Can you work these out from the model? Positions are in its coordinate system, mm. A direction names the side the tool comes from. Give positions to 0.01 mm unless a question says otherwise; leave off trailing zeros. Order: outer loops, then holes, each group sorted by start corner. A loop starts at its lowest first (then second) coordinate and runs counter-clockwise, first axis right, second up. Notation, with made-up numbers: (85, 71) -> (95, 71) arc R21 ccw to (95, 97) -> close; hole circle Ø9 at (-10, -13.5). An arc over 180 degrees is marked (long way). Answer as a JSON object with one key per item and string values.
```python
from build123d import *

# Parameters (mm, degrees)
SKETCH1_R              = 14.2875
BOSS_EXTRUDE1_DEPTH    = 3.175
SKETCH2_W              = 44.45
SKETCH2_H              = 3.175
BOSS_EXTRUDE2_DEPTH    = 50.8
FILLET1_R              = 2.54
CONVERT_SOLID1_START   = -22.225
CONVERT_SOLID1_DEPTH   = 44.45
CONVERT_SOLID1_2_DEPTH = 44.45
SKETCH7_R              = 2.413
CUT_EXTRUDE1_DEPTH     = 50.8


# Read off the part's stored shape, not the designer's step: Convert-Solid1
with BuildPart() as part:
    # Sketch1 → Boss-Extrude1 (new body)
    with BuildSketch(Plane.XY):
        with BuildLine():
            Line((-22.225, -46.491872792), (22.225, -46.491872792))
            Line((22.225, -46.491872792), (22.225, 43.951872792))
            ThreePointArc((22.225, 43.951872792), (21.481051224, 45.747924016), (19.685, 46.491872792))
            Line((19.685, 46.491872792), (-19.685, 46.491872792))
            ThreePointArc((-19.685, 46.491872792), (-21.481051224, 45.747924016), (-22.225, 43.951872792))
            Line((-22.225, 43.951872792), (-22.225, -46.491872792))
        make_face()
        with Locations((0, 22.596127208)):
            Circle(SKETCH1_R, mode=Mode.SUBTRACT)
    extrude(amount=BOSS_EXTRUDE1_DEPTH)

    # Sketch2 → Boss-Extrude2 (add)
    with BuildSketch(Plane(origin=(0, 0, 0), x_dir=(-1, 0, 0), z_dir=(0, 0, -1))):
        with Locations((0, -44.904372792)):
            Rectangle(SKETCH2_W, SKETCH2_H)
    extrude(amount=BOSS_EXTRUDE2_DEPTH)

    # Fillet1
    fillet1_edges = [part.edges().sort_by_distance(p)[0] for p in [
        (22.225, -44.904372792, -50.8),
        (-22.225, -44.904372792, -50.8),
    ]]
    fillet(fillet1_edges, radius=FILLET1_R)

    # Convert-Solid1 outline → Convert-Solid1 (cut)
    with BuildSketch(Plane.YZ.offset(CONVERT_SOLID1_START)):
        with BuildLine():
            ThreePointArc((-46.491872792, -3.81), (-44.446013659, 1.129140866), (-39.506872792, 3.175))
            Line((-39.506872792, 3.175), (-46.491872792, 3.175))
            Line((-46.491872792, 3.175), (-46.491872792, -3.81))
        make_face()
    extrude(amount=CONVERT_SOLID1_DEPTH, mode=Mode.SUBTRACT)

    # Convert-Solid1 2 outline → Convert-Solid1 2 (add)
    with BuildSketch(Plane.YZ.offset(CONVERT_SOLID1_START)):
        with BuildLine():
            ThreePointArc((-43.316872792, -3.81), (-42.200949628, -1.115923164), (-39.506872792, 0))
            Line((-39.506872792, 0), (-43.316872792, 0))
            Line((-43.316872792, 0), (-43.316872792, -3.81))
        make_face()
    extrude(amount=CONVERT_SOLID1_2_DEPTH)

    # Sketch7 → Cut-Extrude1 (cut)
    with BuildSketch(Plane(origin=(0, -43.316872792, 0), x_dir=(1, 0, 0), z_dir=(0, 1, 0))):
        with Locations(Location((-10.795, 39.37, 0), (0, 0, 180))):
            Circle(SKETCH7_R)
        with Locations(Location((10.795, 39.37, 0), (0, 0, 180))):
            Circle(SKETCH7_R)
        with Locations(Location((-10.795, 16.51, 0), (0, 0, 180))):
            Circle(SKETCH7_R)
        with Locations(Location((10.795, 16.51, 0), (0, 0, 180))):
            Circle(SKETCH7_R)
    extrude(amount=-CUT_EXTRUDE1_DEPTH, mode=Mode.SUBTRACT)


solid = part.part
```
1. For faces 1 (the face through (22.225, -14.9, 0.4)), 2 (the face through (0, 4, 0)), which set-ups out of +Z, -Z, +X, -X, +Y, -Y let a thin tool reach every point of the face, with its end or its side?
Worked answers:
{"face 1": "+Z, -Z, +X, +Y, -Y", "face 2": "-Z, +X, -X, +Y"}
2. Will these pins go through, and if not, where does the flat tip stop? pin 1 Ø10 at (x, z) = (2, -6.5) entering from +Y; pin 2 Ø7.5 at (x, z) = (10.795, -16.51) entering from -Y; pin 3 Ø1 at (x, z) = (-2, -45) entering from +Y.
Worked answers:
{"pin 1": "y = -42.54", "pin 2": "y = -46.49", "pin 3": "y = -43.32"}
3. If we section it at B-B on y = 21.5: Please give me the cut outline in (x, z) (3 decimals), then the cut area to 3 significant figures.
Worked answers:
{"outline": "(-22.225, 0) -> (-14.245, 0) -> (-14.245, 3.175) -> (-22.225, 3.175) -> close; (14.245, 0) -> (22.225, 0) -> (22.225, 3.175) -> (14.245, 3.175) -> close", "area": "50.7 mm²"}
4. If we section it at C-C on x = 0: Please give me the cut outline in (y, z) (3 decimals).
Worked answers:
{"outline": "(-46.492, -50.8) -> (-43.317, -50.8) -> (-43.317, -3.81) arc R3.81 cw to (-39.507, 0) -> (8.309, 0) -> (8.309, 3.175) -> (-39.507, 3.175) arc R6.985 ccw to (-46.492, -3.81) -> close; (36.884, 0) -> (46.492, 0) -> (46.492, 3.175) -> (36.884, 3.175) -> close"}
5. Please list where these lines run through material, in increasing order: L1, parallel to X at y = -44, z = -16 (3 decimals); L2, parallel to Z at x = -6, y = -28 (3 decimals); L3, parallel to Y at x = -12, z = -14.
Worked answers:
{"L1": "-22.225 to -13.153, -8.437 to 8.437, 13.153 to 22.225", "L2": "0 to 3.175", "L3": "-46.49 to -43.32"}
6. If we mould it in two halves opening along Z, with no side actions, what happens to faces 3 (the face through (-21.501, -44.882, -50.036)), 4 (the face through (0, -43.317, -27)), 5 (the face through (12.573, -44.882, -14.879))? For each: +Z half, -Z half, draft (parallel to the pull), parting line (faces both ways), or undercut.
Worked answers:
{"face 3": "-Z half", "face 4": "draft", "face 5": "undercut"}
7. If we section it at D-D on x = 11: Please give me the cut outline in (y, z) (3 decimals).
Worked answers:
{"outline": "(-46.492, -50.8) -> (-43.317, -50.8) -> (-43.317, -41.774) -> (-46.492, -41.774) -> close; (-46.492, -36.966) -> (-43.317, -36.966) -> (-43.317, -18.914) -> (-46.492, -18.914) -> close; (-46.492, -14.106) -> (-43.317, -14.106) -> (-43.317, -3.81) arc R3.81 cw to (-39.507, 0) -> (13.478, 0) -> (13.478, 3.175) -> (-39.507, 3.175) arc R6.985 ccw to (-46.492, -3.81) -> close; (31.714, 0) -> (46.492, 0) -> (46.492, 3.175) -> (31.714, 3.175) -> close"}
8. If we section it at A-A on z = -39.37: Please give me the cut outline in (x, y) (3 decimals).
Worked answers:
{"outline": "(-22.225, -46.492) -> (-13.208, -46.492) -> (-13.208, -43.317) -> (-22.225, -43.317) -> close; (-8.382, -46.492) -> (8.382, -46.492) -> (8.382, -43.317) -> (-8.382, -43.317) -> close; (13.208, -46.492) -> (22.225, -46.492) -> (22.225, -43.317) -> (13.208, -43.317) -> close"}
